```python
from build123d import *

# Parameters (mm, degrees)
SALIENTE_EXTRUIR1_DEPTH = 4.98
CROQUIS2_R              = 1
CORTAR_EXTRUIR1_DEPTH   = 5
CORTAR_EXTRUIR3_REACH   = 36.304
CROQUIS4_R              = 1


with BuildPart() as part:
    # Croquis1 → Saliente-Extruir1 (new body)
    with BuildSketch(Plane.XY):
        with BuildLine():
            Line((0, -4), (0, 26))
            Line((0, 26), (21.816861247, 21.191410261))
            add(Edge.make_bspline(
                [(0, -4), (2.906764931, -3.267903802), (7.189424572, -1.091865696), (11.643736623, 3.460788761), (14.473771474, 7.480841145), (17.337780125, 11.369260365), (19.648075945, 16.032903585), (21.017709919, 19.355582105), (21.816861247, 21.191410261)],
                knots=[0, 0, 0, 0, 0.260017683, 0.40718949, 0.54930604, 0.687276252, 0.826057346, 1, 1, 1, 1], degree=3))
        make_face()
    extrude(amount=SALIENTE_EXTRUIR1_DEPTH)

    # Croquis2 → Cortar-Extruir1 (cut)
    with BuildSketch(Plane.XY.offset(4.98)):
        with Locations((1.5, 21.5)):
            Circle(CROQUIS2_R)
    extrude(amount=-CORTAR_EXTRUIR1_DEPTH, mode=Mode.SUBTRACT)

    # Croquis4 → Cortar-Extruir3 (cut, up to next)
    with BuildSketch(Plane.XY.offset(4.98), mode=Mode.PRIVATE) as cortar_extruir3_sk1:
        with Locations((1.216735104, 3.291060379)):
            Circle(CROQUIS4_R)
    cortar_extruir3_tool1 = extrude(cortar_extruir3_sk1.sketch, amount=-CORTAR_EXTRUIR3_REACH, mode=Mode.PRIVATE) & part.part
    add(cortar_extruir3_tool1.solids().sort_by_distance((1.216735, 3.29106, 4.98))[0], mode=Mode.SUBTRACT)


solid = part.part
```
Verification items for the finished model (mm, model axes). Give positions to 0.01 mm unless a question says otherwise; leave off trailing zeros. Order: outer loops, then holes, each group sorted by start corner. A loop starts at its lowest first (then second) coordinate and runs counter-clockwise, first axis right, second up. Notation, with made-up numbers: (-39.75, -16) -> (18.25, -16) arc R28 cw to (18.25, 9) -> close; hole circle Ø5 at (20.5, -35.75). An arc over 180 degrees is marked (long way). One line per item, written item: value.
(1) Sectioned sample at A-A on y = 21.5. Record the cut outline in (x, z).
Final values:
outline: (0, 0) -> (0.5, 0) -> (0.5, 4.98) -> (0, 4.98) -> close; (2.5, 0) -> (20.42, 0) -> (20.42, 4.98) -> (2.5, 4.98) -> close
(2) Draft check along Y on faces 1 (the face through (0.48, 3.97, 2.52)), 2 (the face through (9, 11, 4.98)), 3 (the face through (10.76, 23.63, 2.46)). Enter one of: pulls with the +Y half, pulls with the -Y half, needs draft (parallel to the pull), parting line crosses it, or undercut.
Final values:
face 1: undercut
face 2: needs draft
face 3: pulls with the +Y half
(3) Scan lines: line 1 along Y through (x, z) = (1.5, 3.25); line 2 along Y through (x, z) = (20, 3.15); line 3 along Y through (x, z) = (13, 0.9). Record each from-to range of solid material in increasing order. Write a range as [from, to].
Final values:
line 1: [-3.56, 2.33], [4.25, 20.5], [22.5, 25.67]
line 2: [16.98, 21.59]
line 3: [5.42, 23.13]
(4) Sectioned sample at B-B on x = 1.5. Count the separate pieces of the cut face and the enclosed holes in it, then the cut area to 3 significant figures.
Final values:
separate pieces: 3
enclosed holes: 0
area: 126 mm^2
(5) Gauge pin test, flat ends, axial feed: pin 1 (1 mm diameter, centred on x = 2, z = 3, fed in from -Y); pin 2 (8 mm diameter, centred on x = 10, y = 9.5, fed in from -Z); pin 3 (1 mm diameter, centred on x = 4.5, z = 0.5, fed in from +Y). Record the tip position at first contact, or that the pin passes through.
Final values:
pin 1: y = -3.56
pin 2: z = 0
pin 3: y = 25.12
